```python
from build123d import *

# Parameters (mm, degrees)
SKETCH_3_W          = 70
SKETCH_3_H          = 5
EXTRUDE_3_DEPTH     = 15
CUT_EXTRUDE_1_REACH = 73.764
SKETCH_4_R          = 2
SKETCH_7_W          = 40
SKETCH_7_H          = 15
EXTRUDE_5_DEPTH     = 2
CUT_EXTRUDE_2_REACH = 80.147
SKETCH_9_R          = 1.6


with BuildPart() as part:
    # 草图3 → 凸台-拉伸3 (new body)
    with BuildSketch(Plane.XY):
        with Locations((35, 2.5)):
            Rectangle(SKETCH_3_W, SKETCH_3_H)
    extrude(amount=EXTRUDE_3_DEPTH)

    # 草图4 → 切除-拉伸1 (cut, up to next)
    with BuildSketch(Plane(origin=(0, 0, 0), x_dir=(1, 0, 0), z_dir=(0, 1, 0)), mode=Mode.PRIVATE) as cut_extrude_1_sk1:
        with Locations((5.878824242, -7.5)):
            Circle(SKETCH_4_R)
    cut_extrude_1_tool1 = extrude(cut_extrude_1_sk1.sketch, amount=CUT_EXTRUDE_1_REACH, mode=Mode.PRIVATE) & part.part
    add(cut_extrude_1_tool1.solids().sort_by_distance((5.878824, 0, 7.5))[0], mode=Mode.SUBTRACT)

    # 草图7 → 凸台-拉伸5 (add)
    with BuildSketch(Plane(origin=(70, 0, 0), x_dir=(0, 0, -1), z_dir=(1, 0, 0))):
        with Locations((-7.494082881, 5.421691662)):
            Rectangle(SKETCH_7_W, SKETCH_7_H)
    extrude(amount=EXTRUDE_5_DEPTH)

    # 草图9 → 切除-拉伸2 (cut, up to next)
    with BuildSketch(Plane(origin=(72, 0, 0), x_dir=(0, 0, -1), z_dir=(1, 0, 0)), mode=Mode.PRIVATE) as cut_extrude_2_sk1:
        with Locations((-21.210082881, 9.92331395)):
            Circle(SKETCH_9_R)
    cut_extrude_2_tool1 = extrude(cut_extrude_2_sk1.sketch, amount=-CUT_EXTRUDE_2_REACH, mode=Mode.PRIVATE) & part.part
    # 草图9 → 切除-拉伸2 (cut, up to next)
    with BuildSketch(Plane(origin=(72, 0, 0), x_dir=(0, 0, -1), z_dir=(1, 0, 0)), mode=Mode.PRIVATE) as cut_extrude_2_sk2:
        with Locations((6.221917119, 9.92331395)):
            Circle(SKETCH_9_R)
    cut_extrude_2_tool2 = extrude(cut_extrude_2_sk2.sketch, amount=-CUT_EXTRUDE_2_REACH, mode=Mode.PRIVATE) & part.part
    add(cut_extrude_2_tool1.solids().sort_by_distance((72, 9.923314, 21.210083))[0], mode=Mode.SUBTRACT)
    add(cut_extrude_2_tool2.solids().sort_by_distance((72, 9.923314, -6.221917))[0], mode=Mode.SUBTRACT)


solid = part.part
```
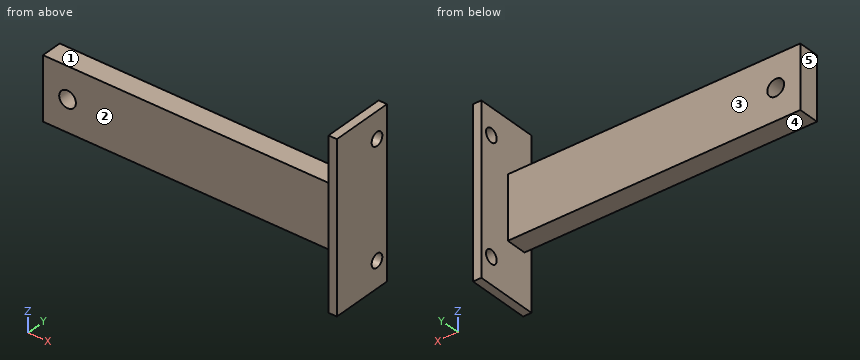
Read the model definition and answer for the solid it produces. Units are mm, in the model's axes. Face numbers are marked on the shaded views. A direction names the side the tool comes from. Coordinates: 2 decimals unless noted, no trailing zeros. Write each loop counter-clockwise with the first axis right and the second up, starting at its lowest first coordinate (ties: lowest second). Pieces come first, ordered by that corner, then holes. Notation, with made-up numbers: (36.5, 44) -> (82.5, 44) arc R18 cw to (82.5, 52) -> close; hole circle Ø6 at (49, 3.25). An arc over 180 degrees is marked (long way). Return JSON: item names as keys, results as strings.
1. A cutting plane is placed at D-D (z = 1). Determine the outline of the cut face in (x, y).
Found:
{"outline": "(0, 0) -> (70, 0) -> (70, -2.08) -> (72, -2.08) -> (72, 12.92) -> (70, 12.92) -> (70, 5) -> (0, 5) -> close"}
2. A cutting plane is placed at C-C (x = 6). Determine the outline of the cut face in (y, z).
Found:
{"outline": "(0, 0) -> (5, 0) -> (5, 5.5) -> (0, 5.5) -> close; (0, 9.5) -> (5, 9.5) -> (5, 15) -> (0, 15) -> close"}
3. A tool of negligible diameter and unlimited length cuts with its end or side. For the marked faces 1, 2, 3, 4 and 5, from which of +Z, -Z, +X, -X, +Y, -Y can it reach the whole face along a straight path? Write none if from no direction.
Found:
{"face 1": "+Z, -X, +Y, -Y", "face 2": "+Z, -Z, -X, -Y", "face 3": "+Z, -Z, -X, +Y", "face 4": "-Z, -X, +Y, -Y", "face 5": "+Z, -Z, -X, +Y, -Y"}
4. A cutting plane is placed at A-A (y = 1.75). Determine the outline of the cut face in (x, z).
Found:
{"outline": "(0, 0) -> (70, 0) -> (70, -12.51) -> (72, -12.51) -> (72, 27.49) -> (70, 27.49) -> (70, 15) -> (0, 15) -> close; hole circle Ø4 at (5.88, 7.5)"}
5. Each of these flat-tipped pins is pushed along its axis until it touches: P1, Ø5, axis at x = 25.5, z = 14.5, coming from the +Y side; P2, Ø5.5, axis at x = 28.5, y = 3, coming from the -Z side; P3, Ø6.5, axis at x = 5.88, z = 7.5, coming from the -Y side. Where does it stop, or does it pass through?
Found:
{"P1": "y = 5", "P2": "z = 0", "P3": "y = 0"}
6. Find the intervals of material crossed by line 1 along X through (y, z) = (2.65, 7.5); line 2 along X through (y, z) = (7.5, -10); line 3 along Z through (x, y) = (44.5, 3), in increasing order. Write a range as from..to.
Found:
{"line 1": "0..3.88, 7.88..72", "line 2": "70..72", "line 3": "0..15"}
7. A cutting plane is placed at B-B (z = 7.5). Determine the outline of the cut face in (x, y).
Found:
{"outline": "(0, 0) -> (3.88, 0) -> (3.88, 5) -> (0, 5) -> close; (7.88, 0) -> (70, 0) -> (70, -2.08) -> (72, -2.08) -> (72, 12.92) -> (70, 12.92) -> (70, 5) -> (7.88, 5) -> close"}
